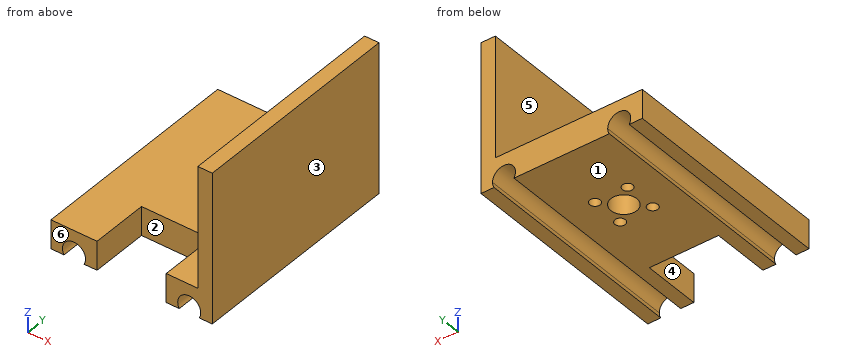
```python
from build123d import *

# Parameters (mm, degrees)
F0_W     = 56
F0_H     = 75
F0_R     = 1.8
F0_R_2   = 4.5
F1_DEPTH = 10
F3_DEPTH = 75.001
F4_W     = 24
F4_H     = 20
F5_DEPTH = 25
F6_W     = 5
F6_H     = 75
F7_DEPTH = 42


with BuildPart() as f1:
    # F0 (on Top) → F1 (new body)
    with BuildSketch(Plane.XY):
        Rectangle(F0_W, F0_H)
        with Locations((-5.6568542495, 3.8431457505)):
            Circle(F0_R, mode=Mode.SUBTRACT)
        with Locations((-5.6568542495, 15.1568542495)):
            Circle(F0_R, mode=Mode.SUBTRACT)
        with Locations((5.6568542495, 3.8431457505)):
            Circle(F0_R, mode=Mode.SUBTRACT)
        with Locations((0, 9.5)):
            Circle(F0_R_2, mode=Mode.SUBTRACT)
        with Locations((5.6568542495, 15.1568542495)):
            Circle(F0_R, mode=Mode.SUBTRACT)
    extrude(amount=F1_DEPTH)

    # F2 (on face) → F3 (cut, through all)
    with BuildSketch(Plane.XZ.offset(37.5)):
        with BuildLine():
            ThreePointArc((-16.5358983849, 0), (-16.1362966948, 0.9647238196), (-16, 2))
            ThreePointArc((-16, 2), (-21.0352761804, 5.8637033052), (-23.4641016151, 0))
            Line((-23.4641016151, 0), (-16.5358983849, 0))
        make_face()
        with BuildLine():
            ThreePointArc((24, 2), (18.9647238196, 5.8637033052), (16.5358983849, 0))
            Line((16.5358983849, 0), (23.4641016151, 0))
            ThreePointArc((23.4641016151, 0), (23.8637033052, 0.9647238196), (24, 2))
        make_face()
    extrude(amount=-F3_DEPTH, mode=Mode.SUBTRACT)

    # F4 (on face) → F5 (cut)
    with BuildSketch(Plane.XY.offset(10)):
        with Locations((0, -27.5)):
            Rectangle(F4_W, F4_H)
    extrude(amount=-F5_DEPTH, mode=Mode.SUBTRACT)

    # F6 (on face) → F7 (join)
    with BuildSketch(Plane.XY.offset(10)):
        with Locations((25.5, 0)):
            Rectangle(F6_W, F6_H)
    extrude(amount=F7_DEPTH)


solid = f1.part
```
Geometry: final body of the model. Coordinates: model frame, mm. Face numbers are marked on the shaded views. A direction names the side the tool comes from. Round coordinates to 2 decimals unless told otherwise and drop trailing zeros. Order: outer loops, then holes, each group sorted by start corner. A loop starts at its lowest first (then second) coordinate and runs counter-clockwise, first axis right, second up. Notation, with made-up numbers: M 77,52 L 121,52 A23 cw 121,60 Z; hole C -21,61 d1. An arc over 180 degrees is marked long. Use one line per item in the form item = value. Start each with the question number.
Q1. Cut plane A-A (x = 0). Return loops of the section in (y, z).
Q2. Mould query, pull axis X, two halves, no side actions, for the marked faces 1, 2 and 3. Classes: +X half, -X half, draft (parallel to the pull), parting line (faces both ways), or undercut.
Q3. Cut plane D-D (z = 42). Return loops of the section in (x, y), and give its area (3 significant figures).
Q4. Access query for the marked faces 4, 5 and 6. Directions: +Z, -Z, +X, -X, +Y, -Y. A direction counts if a zero-diameter tool reaches every point of the face in a straight line with its end or side. Return the directions, or none.
Q5. Pin query (flat end, axial travel): pin 1 Ø6 at (x, y) = (5.66, 3.84) entering from +Z; pin 2 Ø21 at (y, z) = (15.5, 35) entering from -X; pin 3 Ø6 at (x, z) = (1, 8.5) entering from -Y. Return the tip coordinate at first contact, or that it passes through.
Q6. Material intervals for line 1 (X direction, y = 15, z = 2); line 2 (X direction, y = -21, z = 3.5); line 3 (Y direction, x = -7, z = 3), sorted ascending. Write a range as [from, to].
Q7. Cut plane C-C (y = -11). Return loops of the section in (x, z).
Q8. Cut plane B-B (y = -22.5). Return loops of the section in (x, z).
Geometry results:
q1.outline = M -17.5,0 L 5,0 L 5,10 L -17.5,10 Z; M 14,0 L 37.5,0 L 37.5,10 L 14,10 Z
q2.face_1 = draft
q2.face_2 = undercut
q2.face_3 = +X half
q3.outline = M 23,-37.5 L 28,-37.5 L 28,37.5 L 23,37.5 Z
q3.area = 375 mm^2
q4.face_4 = +Z, -Z, -Y
q4.face_5 = +Z, -X, +Y, -Y
q4.face_6 = +Z, -Z, +X, -X, -Y
q5.pin_1 = 10
q5.pin_2 = 23
q5.pin_3 = -17.5
q6.line_1 = [-28, -24], [-16, -7.45], [-3.86, 3.86], [7.45, 16], [24, 28]
q6.line_2 = [-28, -23.71], [-16.29, -12], [12, 16.29], [23.71, 28]
q6.line_3 = [-17.5, 2.64], [5.04, 13.96], [16.36, 37.5]
q7.outline = M -28,0 L -23.46,0 A4 cw long -16.54,0 L 16.54,0 A4 cw long 23.46,0 L 28,0 L 28,52 L 23,52 L 23,10 L -28,10 Z
q8.outline = M -28,0 L -23.46,0 A4 cw long -16.54,0 L -12,0 L -12,10 L -28,10 Z; M 12,0 L 16.54,0 A4 cw long 23.46,0 L 28,0 L 28,52 L 23,52 L 23,10 L 12,10 Z
